Read the model definition and answer for the solid it produces. Units are mm, in the model's axes. Face numbers are marked on the shaded views. A direction names the side the tool comes from. Coordinates: 2 decimals unless noted, no trailing zeros. Write each loop counter-clockwise with the first axis right and the second up, starting at its lowest first coordinate (ties: lowest second). Pieces come first, ordered by that corner, then holes.
(1) Straight lines are drawn through the part: line 1 along Y through (x, z) = (0, 8); line 2 along Z through (x, y) = (-3.25, 5); line 3 along Z through (x, y) = (1.5, -1.5). For each, find the intervals that lie inside material, in ascending order.
(2) Given pin 1 (1.5 mm diameter, centred on y = -3.5, z = 111, fed in from +X); pin 2 (1.5 mm diameter, centred on x = -1.5, z = 90, fed in from +Y); pin 3 (8 mm diameter, centred on y = 0, z = 89.5, fed in from -X), each flat-ended and moving along its own axis, determine where each tip first touches the part or whether it passes through.
(3) The part is cut by section B-B, the plane z = 28. Determine the outline of the cut face in (x, y), and give its area (3 significant figures).
(4) The part is cut by section A-A, the plane x = 0. Determine the outline of the cut face in (y, z).
(5) Which of the six approach directions +Z, -Z, +X, -X, +Y, -Y give full straight-line access (tool end or side, diameter ignored) to the marked faces 1 and 2?
(6) The part is cut by section C-C, the plane z = 104.5. Determine the outline of the cut face in (x, y), and give its area (3 significant figures).
```python
from build123d import *

# Parameters (mm, degrees)
F2_W     = 19.6017324924
F2_H     = 37.1457748115
F2_W_2   = 14
F2_H_2   = 30
F3_DEPTH = 8
F4_SIZE  = 0.99999


# Not quite as in the source:
# - a fillet or chamfer is up to 0.001 mm smaller than in the source, because OpenCascade refuses the exact size


with BuildPart() as f1:
    # F0 (on Front) → F1 (revolve)
    with BuildSketch(Plane.XZ):
        with BuildLine():
            Line((2.9315422289, 21.0469197482), (2.9315422289, 0))
            Line((2.9315422289, 0), (8, 0))
            Line((8, 0), (8, 10.8380244002))
            ThreePointArc((8, 10.8380244002), (7.5, 11.3380244002), (8, 11.8380244002))
            Line((8, 11.8380244002), (8, 30.5))
            Line((8, 30.5), (5, 30.5))
            Line((5, 30.5), (5, 130.5))
            Line((5, 130.5), (0, 130.5))
            Line((0, 130.5), (0, 30.5))
            Line((0, 30.5), (0, 21.0469197482))
            Line((0, 21.0469197482), (2.9315422289, 21.0469197482))
        make_face()
    revolve(axis=Axis((0, 0, 80.5), (0, 0, 1)))

    # F2 (on face) → F3 (cut)
    with BuildSketch(Plane.XY.offset(30.5)):
        Rectangle(F2_W, F2_H)
        Rectangle(F2_W_2, F2_H_2, mode=Mode.SUBTRACT)
    extrude(amount=-F3_DEPTH, mode=Mode.SUBTRACT)

    # F4 (size 1 in the source; OpenCascade refuses exactly that, so slightly less here)
    f4_edges = [f1.edges().sort_by_distance(p)[0] for p in [
        (-7, 0, 22.5),
        (7, 0, 22.5),
    ]]
    chamfer(f4_edges, length=F4_SIZE)


solid = f1.part
```
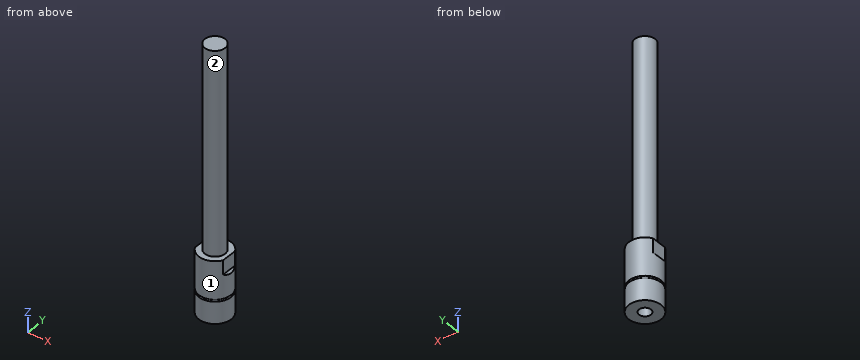
Computed:
1. line 1: y = -8 to -2.93, 2.93 to 8
1. line 2: z = 0 to 30.5
1. line 3: z = 21.05 to 130.5
2. pin 1: stops at x = 4.18
2. pin 2: stops at y = 4.94
2. pin 3: stops at x = -5
3. outline: (-7, -3.87) arc R8 ccw to (7, -3.87) - (7, 3.87) arc R8 ccw to (-7, 3.87) - close
3. area: 191 mm2
4. outline: (-8, 0) - (-2.93, 0) - (-2.93, 21.05) - (2.93, 21.05) - (2.93, 0) - (8, 0) - (8, 10.84) arc R0.5 cw to (8, 11.84) - (8, 30.5) - (5, 30.5) - (5, 130.5) - (-5, 130.5) - (-5, 30.5) - (-8, 30.5) - (-8, 11.84) arc R0.5 cw to (-8, 10.84) - close
5. face 1: +Z, -Z
5. face 2: +Z
6. outline: circle Ø10 at (0, 0)
6. area: 78.5 mm2
